For this review, take the finished solid that the model builds, in its own axes (mm). A direction names the side the tool comes from. Round coordinates to 2 decimals unless told otherwise and drop trailing zeros. Write each loop counter-clockwise with the first axis right and the second up, starting at its lowest first coordinate (ties: lowest second). Pieces come first, ordered by that corner, then holes. Notation, with made-up numbers: (46, 79.5) -> (85, 79.5) arc R23 cw to (85, 109.5) -> close; hole circle Ø3 at (-34.75, 72.5). An arc over 180 degrees is marked (long way). Answer in a Markdown table with one row per item. Add a question column.
```python
from build123d import *

# Parameters (mm, degrees)
CROQUIS1_W              = 30
CROQUIS1_H              = 33
SALIENTE_EXTRUIR1_DEPTH = 22
CHAFL_N1_SIZE           = 5
CHAFL_N2_SIZE           = 5
CROQUIS3_R              = 2
CORTAR_EXTRUIR1_DEPTH   = 35
CROQUIS2_R              = 2
SALIENTE_EXTRUIR2_DEPTH = 5


with BuildPart() as part:
    # Croquis1 → Saliente-Extruir1 (new body)
    with BuildSketch(Plane.XY):
        with Locations((-0.166051661, -4.433579336)):
            Rectangle(CROQUIS1_W, CROQUIS1_H)
    extrude(amount=SALIENTE_EXTRUIR1_DEPTH)

    # Chaflán1
    chafl_n1_edges = [part.edges().sort_by_distance(p)[0] for p in [
        (-0.166051661, 12.066420664, 0),
    ]]
    chamfer(chafl_n1_edges, length=CHAFL_N1_SIZE)

    # Chaflán2
    chafl_n2_edges = [part.edges().sort_by_distance(p)[0] for p in [
        (-0.166051661, -20.933579336, 0),
    ]]
    chamfer(chafl_n2_edges, length=CHAFL_N2_SIZE)

    # Croquis3 → Cortar-Extruir1 (cut)
    with BuildSketch(Plane(origin=(14.833948339, 0, 0), x_dir=(0, 0, -1), z_dir=(1, 0, 0))):
        with Locations(Location((-12, 2.066420664, 0), (0, 0, 90))):
            Circle(CROQUIS3_R)
    extrude(amount=-CORTAR_EXTRUIR1_DEPTH, mode=Mode.SUBTRACT)

    # Croquis2 → Saliente-Extruir2 (add)
    with BuildSketch(Plane.XY.offset(22)):
        with Locations((-0.166051661, -10.933579336)):
            Circle(CROQUIS2_R)
    extrude(amount=SALIENTE_EXTRUIR2_DEPTH)


solid = part.part
```
1. We need section A-A (x = -10). Write out the cut boundary in (y, z).
2. Clearance check with flat-ended pins moving along their axes: pin 1 Ø2.5 at (y, z) = (2.07, 12) entering from +X; pin 2 Ø1.5 at (x, y) = (-3, -6) entering from +Z. State where each tip first meets the part, or that it passes through.
3. The part is to be moulded in two halves that separate along Z. For faces 3 (the flat face through (0, -11, 27)), 4 (the cylindrical face through (0, 2, 14)), 5 (the flat face through (-15.166, -5, 11)), say which applies: pulls with the +Z half, pulls with the -Z half, needs draft (parallel to the pull), parting line crosses it, or undercut.
4. We need section D-D (y = -14). Write out the cut boundary in (x, z).
5. Tool access review of faces 1 (the flat face through (14.834, -5, 11)), 2 (the cylindrical face through (-0.43, -8.95, 24.46)): name each direction out of +Z, -Z, +X, -X, +Y, -Y from which nothing blocks a thin tool from reaching the whole face with its end or side.
6. For L1, parallel to Z at x = 9, y = -13; L2, parallel to Z at x = 8.5, y = 0.5; L3, parallel to Z at x = -5.25, y = 1, list the stretches that pass through material, from the lowest coordinate up. Write a range as [from, to].
7. We need section C-C (y = 1.5). Write out the cut boundary in (x, z).
8. We need section B-B (z = 12). Write out the cut boundary in (x, y), plus the area to 3 significant figures.
Response:
| question | item | result |
|---|---|---|
| 1 | outline | (-20.93, 5) -> (-15.93, 0) -> (7.07, 0) -> (12.07, 5) -> (12.07, 22) -> (-20.93, 22) -> close; hole circle Ø4 at (2.07, 12) |
| 2 | pin 1 | through |
| 2 | pin 2 | z = 22 |
| 3 | face 3 | pulls with the +Z half |
| 3 | face 4 | undercut |
| 3 | face 5 | needs draft |
| 4 | outline | (-15.17, 0) -> (14.83, 0) -> (14.83, 22) -> (-15.17, 22) -> close |
| 5 | face 1 | +Z, -Z, +X, +Y, -Y |
| 5 | face 2 | +Z |
| 6 | L1 | [0, 22] |
| 6 | L2 | [0, 10.76], [13.24, 22] |
| 6 | L3 | [0, 10.31], [13.69, 22] |
| 7 | outline | (-15.17, 0) -> (14.83, 0) -> (14.83, 10.08) -> (-15.17, 10.08) -> close; (-15.17, 13.92) -> (14.83, 13.92) -> (14.83, 22) -> (-15.17, 22) -> close |
| 8 | outline | (-15.17, -20.93) -> (14.83, -20.93) -> (14.83, 0.07) -> (-15.17, 0.07) -> close; (-15.17, 4.07) -> (14.83, 4.07) -> (14.83, 12.07) -> (-15.17, 12.07) -> close |
| 8 | area | 870 mm2 |
